Geometry: see drawing. Coordinates: mm, zero at the bounding-box minimum. A direction names the side the tool comes from. Coordinates: 2 decimals unless noted, no trailing zeros. Order: outer loops, then holes, each group sorted by start corner. A loop starts at its lowest first (then second) coordinate and runs counter-clockwise, first axis right, second up. Notation, with made-up numbers: (-16, 34.5) -> (-9, 34.5) arc R13 ccw to (-9, 59.5) -> close; hole circle Ø4 at (86.25, -6.5). An arc over 180 degrees is marked (long way). Write each question's results on one line, items separated by ' | '.
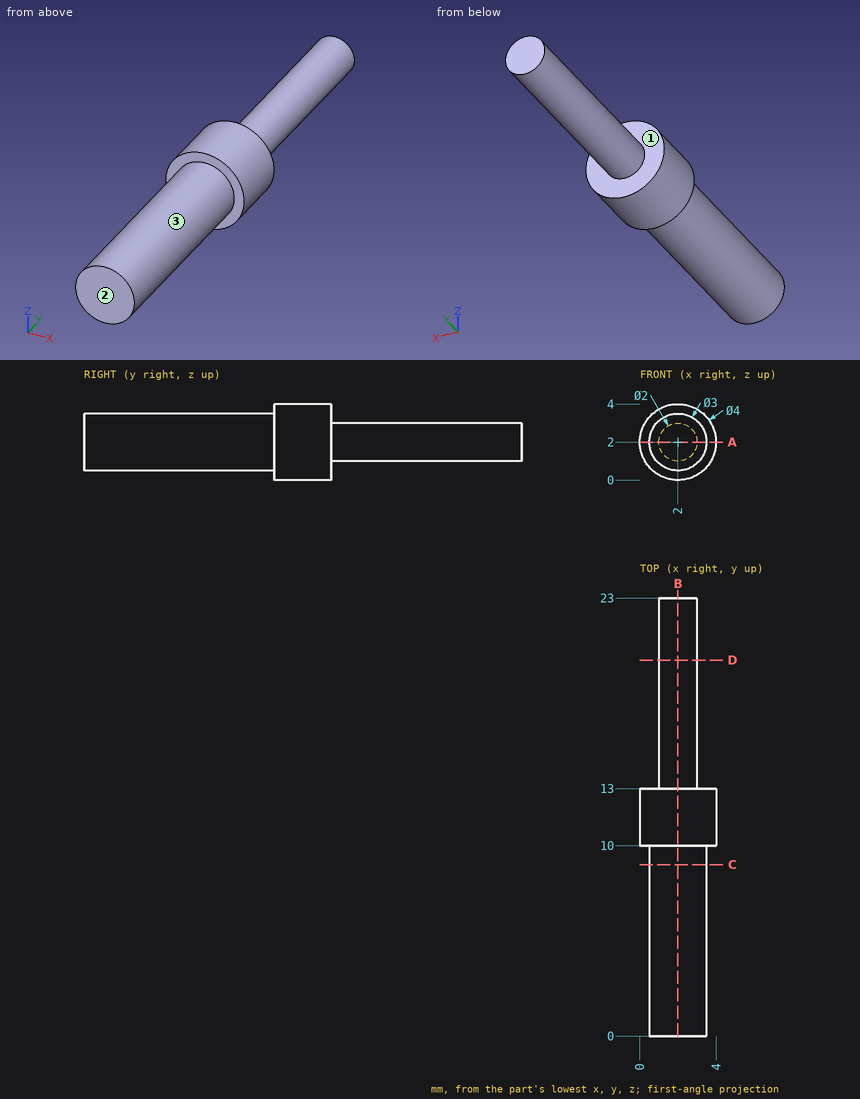
(1) Cut plane D-D, the plane y = 19.75. Return loops of the section in (x, z).
Return value:
outline: circle Ø2 at (2, 2)
(2) Cut plane B-B, the plane x = 2. Return loops of the section in (y, z).
Return value:
outline: (0, 0.5) -> (10, 0.5) -> (10, 0) -> (13, 0) -> (13, 1) -> (23, 1) -> (23, 3) -> (13, 3) -> (13, 4) -> (10, 4) -> (10, 3.5) -> (0, 3.5) -> close
(3) Line query: line 1 along Y through (x, z) = (3.65, 1.4); line 2 along Y through (x, z) = (2.55, 0.8); line 3 along Z through (x, y) = (2.1, 3.5). Output: solid intervals per line, ascending. Write a range as from..to.
Return value:
line 1: 10..13 | line 2: 0..13 | line 3: 0.5..3.5
(4) Reachability of the marked faces 1, 2 and 3 from +Z, -Z, +X, -X, +Y, -Y: full face, straight path, thin tool, end or side. Return the list, or none.
Return value:
face 1: +Y | face 2: +Z, -Z, +X, -X, -Y | face 3: -Y
(5) Cut plane C-C, the plane y = 9. Return loops of the section in (x, z), plus the area to 3 significant figures.
Return value:
outline: circle Ø3 at (2, 2) | area: 7.07 mm2
(6) Cut plane A-A, the plane z = 2. Return loops of the section in (x, y).
Return value:
outline: (0, 10) -> (0.5, 10) -> (0.5, 0) -> (3.5, 0) -> (3.5, 10) -> (4, 10) -> (4, 13) -> (3, 13) -> (3, 23) -> (1, 23) -> (1, 13) -> (0, 13) -> close
